Autodesk Fusion 360 part; units mm, degrees
sketch "Sketch1" plane through (0, 0, 0) normal (0, 1, 0) x (1, 0, 0)
  line L0 (0, 0) -> (12, 0)
  line L1 (0, 0) -> (0, -10)
  line L2 (12, 0) -> (12, -10)
  line L3 (12, -10) -> (0, -10)
  line L4 (12, -10) -> (9, -10)
  arc A0 (9, -10) -> (9, 0) centre (6.3333, -5) ccw
  line L5 (0, -10) -> (3, -10)
  arc A1 (3, 0) -> (3, -10) centre (5.6667, -5) ccw
  dimension "d3" = 12
  dimension "d4" = 10
  dimension "d5" = 3
  dimension "d6" = 3
extrude "Extrude1" add sketch "Sketch1" along normal blind 15.2 contours L0 L3 A0 A1 makes body 1
sketch "Sketch2" plane through (0, 0, 0) normal (0, -1, 0) x (1, 0, 0)
  arc A0 (9, 0) -> (9, 10) centre (6.3333, 5) ccw
  line L0 (9, 10) -> (3, 10)
  arc A1 (3, 10) -> (3, 0) centre (5.6667, 5) ccw
  line L1 (3, 0) -> (9, 0)
  line L2 (0, 10) -> (12, 10)
  line L3 (12, 10) -> (12, 0)
  line L4 (12, 0) -> (0, 0)
  line L5 (0, 0) -> (0, 10)
extrude "Extrude2" add sketch "Sketch2" along normal blind 0.8 bodies 1
sketch "Sketch3" plane through (0, -0.8, 0) normal (0, -1, 0) x (1, 0, 0)
  line L0 (0, 0) -> (12, 0)
  line L1 (12, 0) -> (12, 10)
  line L2 (12, 10) -> (0, 10)
  line L3 (0, 10) -> (0, 0)
  circle A0 centre (2, 2) radius 1.5
  circle A1 centre (10, 8) radius 1.5
  dimension "d11" = 3
  dimension "d12" = 3
extrude "Extrude3" add sketch "Sketch3" along normal blind 2.45 contours A0 | A1 bodies 1
sketch "Sketch4" plane through (0, -3.25, 0) normal (0, -1, 0) x (1, 0, 0)
  circle A0 centre (2, 2) radius 1.5
  line L0 (0, 10) -> (12, 10)
  line L1 (12, 10) -> (12, 0)
  line L2 (12, 0) -> (0, 0)
  line L3 (0, 0) -> (0, 10)
extrude "Extrude4" add sketch "Sketch4" along normal blind 0.8 separate body makes body 2
extrude "Extrude5" add 1 faces at (1.5, -3.25, 2.6802) along direction (0, -1, 0) blind 0.8 on bodies 1 bodies 1 2
sketch "Sketch5" plane through (0, -4.05, 0) normal (0, -1, 0) x (1, 0, 0)
  line L0 (0, 0) -> (12, 0)
  line L1 (12, 0) -> (12, 10)
  line L2 (12, 10) -> (0, 10)
  line L3 (0, 10) -> (0, 0)
  circle A0 centre (2, 2) radius 1.5
  circle A1 centre (10, 8) radius 1.5
  dimension "d19" = 3
  dimension "d20" = 3
extrude "Extrude6" add sketch "Sketch5" along normal blind 4.2 contours A0 | A1 bodies 1
sketch "Sketch6" plane through (0, -8.25, 0) normal (0, -1, 0) x (1, 0, 0)
  circle A0 centre (10, 8) radius 1.5
  line L0 (0, 10) -> (12, 10)
  line L1 (12, 10) -> (12, 0)
  line L2 (12, 0) -> (0, 0)
  line L3 (0, 0) -> (0, 10)
extrude "Extrude7" add sketch "Sketch6" along normal blind 0.8 contours A0 | L0 L1 L2 L3 bodies 1
sketch "Sketch7" plane through (0, -9.05, 0) normal (0, -1, 0) x (1, 0, 0)
  line L0 (0, 0) -> (12, 0)
  line L1 (12, 0) -> (12, 10)
  line L2 (12, 10) -> (0, 10)
  line L3 (0, 10) -> (0, 0)
  line L4 (0, 5) -> (12, 5)
  line L5 (6, 10) -> (6, 0)
  circle A0 centre (6, 5) radius 2.25
  circle A1 centre (0.5, 5) radius 0.35
  circle A2 centre (11.5, 5) radius 0.35
  dimension "d25" = 4.5
  dimension "d26" = 0.7
extrude "Extrude8" cut sketch "Sketch7" against normal blind 2 contours L4 A1 | L4 A1 | L4 A2 | L4 A2 bodies 1
extrude "Extrude9" add sketch "Sketch7" along normal blind 0.87 contours L4 L5 A0 | L4 L5 A0 | L4 L5 A0 | L4 L5 A0 bodies 1
sketch "Sketch8" plane through (0, -9.92, 0) normal (0, -1, 0) x (1, 0, 0)
  circle A0 centre (6, 5) radius 2.25
  line L0 (7.5, 5) -> (5, 5)
  line L1 (5, 5) -> (5, 6.118)
  line L2 (5, 5) -> (5, 3.882)
  arc A1 (5, 3.882) -> (5, 6.118) centre (6, 5) ccw
  dimension "d31" = 3
  dimension "d32" = 2.5
extrude "Extrude10" add sketch "Sketch8" along normal blind 9.17 contours L0 L2 A1 | L0 L1 A1 bodies 1
sketch "Sketch9" plane through (0, 15.2, 0) normal (0, 1, 0) x (-1, 0, 0)
  arc A0 (-9, 10) -> (-9, 0) centre (-6.3333, 5) ccw
  line L0 (-9, 0) -> (-3, 0)
  arc A1 (-3, 0) -> (-3, 10) centre (-5.6667, 5) ccw
  line L1 (-3, 10) -> (-9, 10)
  circle A2 centre (-6, 5) radius 2.5
  line L2 (0, 5) -> (-1.5, 5)
  line L3 (-1.5, 5) -> (-1.5, 4)
  line L4 (0, 5) -> (0, 6)
  line L5 (0, 6) -> (-1.5, 6)
  line L6 (-1.5, 6) -> (-1.5, 4)
  line L7 (-1.5, 4) -> (0, 4)
  line L8 (0, 4) -> (0, 6)
  line L9 (-6, 10) -> (-6, 0)
  line L10 (-10.5, 6) -> (-10.5, 4)
  line L11 (-12, 4) -> (-12, 6)
  line L12 (-10.5, 4) -> (-12, 4)
  line L13 (-12, 6) -> (-10.5, 6)
  dimension "d35" = 5
  dimension "d36" = 1.5
  dimension "d37" = 1
  dimension "d38" = 1
extrude "Extrude11" add sketch "Sketch9" along normal blind 0.9 contours A2 L9 | A2 L9 bodies 1
extrude "Extrude12" cut sketch "Sketch9" against normal blind 2.37 contours A0 L10 L12 L13 | A1 L2 L5 L6 | A1 L2 L3 L6 L7 bodies 1
sketch "Sketch10" plane through (0, 15.2, 0) normal (0, 1, 0) x (-1, 0, 0)
  line L0 (-0.0889, 4) -> (-1.5, 4)
  line L1 (-1.5, 4) -> (-1.5, 6)
  line L2 (-1.5, 6) -> (-0.0889, 6)
  arc A0 (-0.0889, 6) -> (-3, 10) centre (-5.6667, 5) ccw
  line L3 (-3, 10) -> (-9, 10)
  arc A1 (-9, 10) -> (-11.9111, 6) centre (-6.3333, 5) ccw
  line L4 (-11.9111, 6) -> (-10.5, 6)
  line L5 (-10.5, 6) -> (-10.5, 4)
  line L6 (-10.5, 4) -> (-11.9111, 4)
  arc A2 (-11.9111, 4) -> (-9, 0) centre (-6.3333, 5) ccw
  line L7 (-9, 0) -> (-3, 0)
  arc A3 (-3, 0) -> (-0.0889, 4) centre (-5.6667, 5) ccw
  circle A4 centre (-6, 5) radius 2.5
  line L8 (-3.5, 5) -> (-2.39, 5)
  line L9 (-2.39, 5) -> (-2.39, 4.25)
  line L10 (-2.39, 4.25) -> (-2.09, 4.25)
  line L11 (-2.09, 4.25) -> (-2.09, 5)
  line L12 (0, 5) -> (-12, 5)
  line L13 (-3.5, 5) -> (-2.39, 5)
  line L14 (-2.39, 5.75) -> (-2.09, 5.75)
  line L15 (-2.09, 5.75) -> (-2.09, 5)
  line L16 (-2.39, 5) -> (-2.39, 5.75)
  line L17 (-6, 10) -> (-6, 0)
  line L18 (-9.61, 5) -> (-9.61, 4.25)
  line L19 (-9.91, 4.25) -> (-9.91, 5)
  line L20 (-9.61, 4.25) -> (-9.91, 4.25)
  line L21 (-12, 5) -> (0, 5)
  line L22 (-9.61, 5.75) -> (-9.91, 5.75)
  line L23 (-9.61, 5) -> (-9.61, 5.75)
  line L24 (-9.91, 5.75) -> (-9.91, 5)
  dimension "d43" = 1.11
  dimension "d44" = 0.75
  dimension "d45" = 0.3
extrude "Extrude13" add sketch "Sketch10" along normal blind 1.31 contours L9 L10 L11 L12 L21 | L12 L14 L15 L16 L21 | L12 L18 L19 L20 L21 | L12 L21 L22 L23 L24 bodies 1
sketch "Sketch11" plane through (2.09, 0, 0) normal (-1, 0, 0) x (0, -1, 0)
  line L0 (-15.2, 4.25) -> (-15.2, 5.75)
  line L1 (-15.2, 5.75) -> (-16.51, 5.75)
  line L2 (-16.51, 5.75) -> (-16.51, 4.25)
  line L3 (-16.51, 4.25) -> (-15.2, 4.25)
  circle A0 centre (-15.8, 5) radius 0.4
extrude "Extrude14" cut sketch "Sketch11" against normal blind 0.7 contours A0 bodies 1
sketch "Sketch12" plane through (9.91, 0, 0) normal (1, 0, 0) x (0, 1, 0)
  line L0 (15.2, 5.75) -> (15.2, 4.25)
  line L1 (15.2, 4.25) -> (16.51, 4.25)
  line L2 (16.51, 4.25) -> (16.51, 5.75)
  line L3 (16.51, 5.75) -> (15.2, 5.75)
  circle A0 centre (15.8, 5) radius 0.4
extrude "Extrude15" cut sketch "Sketch12" against normal blind 0.4 contours A0 bodies 1
fillet "Fillet1" radius 0.4 2 edges at (9.76, 16.51, 4.25) (9.76, 16.51, 5.75) on bodies 1
fillet "Fillet2" radius 0.4 2 edges at (2.24, 16.51, 4.25) (2.24, 16.51, 5.75) on bodies 1
sketch "Sketch13" plane through (0, 16.1, 0) normal (0, 1, 0) x (-1, 0, 0)
  circle A0 centre (-6, 5) radius 2.5
  circle A1 centre (-6, 5) radius 0.93
  dimension "d56" = 1.86
extrude "Extrude16" cut sketch "Sketch13" against normal blind 0.5 contours A1 bodies 1
equation "d5 = ( 12 / 4 ) * 1 mm"
equation "d7 = 16 mm - 0.8 mm"
equation "d44 = ( 1.5 / 2 ) * 1 mm"
Check sheet for the modelled part. Datum: model origin and axes. Units: mm. A direction names the side the tool comes from. Round coordinates to 2 decimals unless told otherwise and drop trailing zeros. Write each loop counter-clockwise with the first axis right and the second up, starting at its lowest first coordinate (ties: lowest second). Pieces come first, ordered by that corner, then holes. Notation, with made-up numbers: (38, 51) - (79, 51) arc R19 ccw to (79, 64) - close; hole circle Ø5 at (57.5, 76). An arc over 180 degrees is marked (long way). Return JSON: item names as keys, results as strings.
Q1. Cross-section at B-B (z = 8). Record the boundary of the cut face in (x, y), then the cut area to 3 significant figures.
Returned:
{"outline": "(0, -9.05) - (12, -9.05) - (12, -8.25) - (11.5, -8.25) - (11.5, -4.05) - (12, -4.05) - (12, -3.25) - (11.5, -3.25) - (11.5, -0.8) - (12, -0.8) - (12, 0) - (11.14, 0) - (11.14, 15.2) - (0.86, 15.2) - (0.86, 0) - (0, 0) - (0, -0.8) - (8.5, -0.8) - (8.5, -3.25) - (0, -3.25) - (0, -4.05) - (8.5, -4.05) - (8.5, -8.25) - (0, -8.25) - close", "area": "205 mm²"}
Q2. Scan lines: L1, parallel to Y at x = 7.25, z = 4; L2, parallel to Y at x = 11, z = 4.75; L3, parallel to Z at x = 9.75, y = 15.8. Record each from-to range of solid material in increasing order. Write a range as from..to.
Returned:
{"L1": "y = -9.92..-8.25, -4.05..-3.25, -0.8..16.1", "L2": "y = -9.05..-8.25, -4.05..-3.25, -0.8..12.83", "L3": "z = 4.25..4.6, 5.4..5.75"}
Q3. Cross-section at C-C (y = -6.5). Record the boundary of the cut face in (x, z), then the cut area to 3 significant figures.
Returned:
{"outline": "circle Ø3 at (2, 2); circle Ø3 at (10, 8)", "area": "14.1 mm²"}
Q4. Cross-section at D-D (y = 5). Record the boundary of the cut face in (x, z).
Returned:
{"outline": "(3, 0) - (9, 0) arc R5.67 ccw to (9, 10) - (3, 10) arc R5.67 ccw to start"}
Q5. Cross-section at A-A (x = 6.5). Record the boundary of the cut face in (y, z), then the cut area to 3 significant figures.
Returned:
{"outline": "(-19.09, 3.59) - (-9.92, 3.59) - (-9.92, 2.81) - (-9.05, 2.81) - (-9.05, 0) - (-8.25, 0) - (-8.25, 10) - (-9.05, 10) - (-9.05, 7.19) - (-9.92, 7.19) - (-9.92, 6.41) - (-19.09, 6.41) - close; (-4.05, 0) - (-3.25, 0) - (-3.25, 10) - (-4.05, 10) - close; (-0.8, 0) - (15.2, 0) - (15.2, 2.55) - (16.1, 2.55) - (16.1, 4.22) - (15.6, 4.22) - (15.6, 5.78) - (16.1, 5.78) - (16.1, 7.45) - (15.2, 7.45) - (15.2, 10) - (-0.8, 10) - close", "area": "209 mm²"}
Q6. Draft check along X on faces 5 (the cylindrical face through (6.685, 15.854, 5.629)), 6 (the flat face through (6, 16.1, 3.9)), 7 (the cylindrical face through (0.89, -2.01, 0.99)), 8 (the flat face through (4.6, -9.05, 7.3)). Enter one of: released by +X, released by -X, zero draft, split by the parting line, or undercut.
Returned:
{"face 5": "undercut", "face 6": "undercut", "face 7": "split by the parting line", "face 8": "zero draft"}
Q7. Access from +Z, -Z, +X, -X, +Y, -Y to the whole of each face (thin tool, end or side, straight path). Record for faces 1 (the flat face through (6, -0.8, 5)), 2 (the flat face through (1, 14, 4)), 3 (the flat face through (1, 0, 9)), 4 (the cylindrical face through (7.5, -14.4, 5)).
Returned:
{"face 1": "none", "face 2": "-X, +Y", "face 3": "+Z, -X, +Y", "face 4": "-Y"}
Q8. Depth check by flat-ended pin: P1, Ø2, axis at x = 3.5, z = 6, coming from the +Y side; P2, Ø1.5, axis at x = 6, z = 5, coming from the +Y side; P3, Ø0.7, axis at y = 15.5, z = 5, coming from the +X side. Enter the tip coordinate at first touch or a pass-through.
Returned:
{"P1": "stops at y = 16.1", "P2": "stops at y = 15.6", "P3": "stops at x = 10.5"}
